from build123d import *

# Parameters (mm, degrees)
BOSS_EXTRUDE1_DEPTH   = 6
SKETCH3_W             = 7.6
SKETCH3_H             = 7.1
SKETCH3_H_2           = 14.9
CUT_EXTRUDE2_DEPTH    = 21.860671783
SKETCH4_W             = 7.6
SKETCH4_H             = 2.5
SKETCH4_W_2           = 5.5
SKETCH4_H_2           = 3.6
CUT_EXTRUDE3_DEPTH    = 21.860671783
FILLET2_R             = 3
F_2_56_TAPPED_HOLE1_D = 1.778
FILLET3_R             = 0.5
F_2_56_TAPPED_HOLE2_D = 1.778
SKETCH19_R            = 0.5
CUT_EXTRUDE6_DEPTH    = 21.860671783


with BuildPart() as part:
    # Sketch1 → Boss-Extrude1 (new body)
    with BuildSketch(Plane(origin=(7.5, 0, 0), x_dir=(0, 0, -1), z_dir=(1, 0, 0))):
        with BuildLine():
            Line((-10.5, 16.997577099), (-10.5, 5.397577099))
            Line((-10.5, 5.397577099), (-2, 5.397577099))
            Line((-2, 5.397577099), (-2, 15.497577099))
            ThreePointArc((-2, 15.497577099), (-1.5, 15.997577099), (-1, 15.497577099))
            Line((-1, 15.497577099), (-1, -2.902422901))
            Line((-1, -2.902422901), (7, -2.902422901))
            Line((7, -2.902422901), (7, 16.997577099))
            Line((7, 16.997577099), (-10.5, 16.997577099))
        make_face()
    extrude(amount=-BOSS_EXTRUDE1_DEPTH)

    # Sketch3 → Cut-Extrude2 (cut, through all)
    with BuildSketch(Plane.ZY.offset(-1.5)):
        with Locations((6.7, 13.947577099)):
            Rectangle(SKETCH3_W, SKETCH3_H)
        with Locations((-3.7, 10.047577099)):
            Rectangle(SKETCH3_W, SKETCH3_H_2)
    extrude(amount=-CUT_EXTRUDE2_DEPTH, mode=Mode.SUBTRACT)

    # Sketch4 → Cut-Extrude3 (cut, through all)
    with BuildSketch(Plane.ZY.offset(-1.5)):
        with Locations((6.7, 9.147577099)):
            Rectangle(SKETCH4_W, SKETCH4_H)
        with Locations((-4.736302331, 0.797577099)):
            Rectangle(SKETCH4_W_2, SKETCH4_H_2)
    extrude(amount=-CUT_EXTRUDE3_DEPTH, mode=Mode.SUBTRACT)

    # Fillet2
    fillet2_edges = [part.edges().sort_by_distance(p)[0] for p in [
        (1.5, 6.647577099, 10.5),
        (7.5, 6.647577099, 10.5),
        (7.5, -1.952422901, -7),
        (1.5, -1.952422901, -7),
    ]]
    fillet(fillet2_edges, radius=FILLET2_R - 0.0001)  # a hair under: the kernel refuses the full size

    # #2-56 Tapped Hole1 (through all)
    with Locations(Plane(origin=(0, 7.897577099, 0), x_dir=(1, 0, 0), z_dir=(0, 1, 0))):
        with Locations((4.5, -8)):
            Hole(F_2_56_TAPPED_HOLE1_D / 2)

    # Fillet3
    fillet3_edges = [part.edges().sort_by_distance(p)[0] for p in [
        (4.5, 2.597577099, 0.1),
        (4.5, 7.897577099, 2.9),
    ]]
    fillet(fillet3_edges, radius=FILLET3_R)

    # #2-56 Tapped Hole2 (through all)
    with Locations(Plane(origin=(0, -1.002422901, 0), x_dir=(1, 0, 0), z_dir=(0, 1, 0))):
        with Locations((4.5, 5)):
            Hole(F_2_56_TAPPED_HOLE2_D / 2)

    # Sketch19 → Cut-Extrude6 (cut, through all)
    with BuildSketch(Plane(origin=(7.5, 0, 0), x_dir=(0, 0, -1), z_dir=(1, 0, 0))):
        with Locations((2.269145043, -0.719580189)):
            Circle(SKETCH19_R)
    extrude(amount=-CUT_EXTRUDE6_DEPTH, mode=Mode.SUBTRACT)


solid = part.part
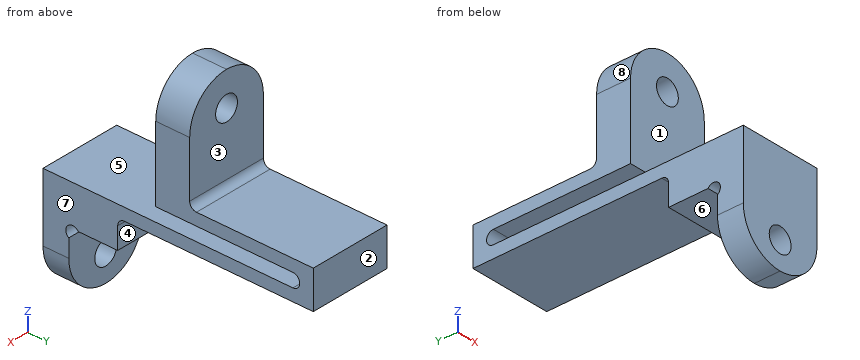
Build history of the part. All positions in model axes, mm. Face numbers are marked on the shaded views. A direction names the side the tool comes from. Round coordinates to 2 decimals unless told otherwise and drop trailing zeros. Write each loop counter-clockwise with the first axis right and the second up, starting at its lowest first coordinate (ties: lowest second). Pieces come first, ordered by that corner, then holes. Notation, with made-up numbers: (-16, 47) -> (-7, 47) arc R14 ccw to (-7, 70) -> close; hole circle Ø8 at (55, 65.25). An arc over 180 degrees is marked (long way). Use one line per item in the form item = value.
Q1. Drill centre lines: L1, parallel to Z at x = 4.5, y = 7.4; L2, parallel to Z at x = 5.5, y = 13; L3, parallel to Y at x = 1.85, z = 2.25. Where is each one in solid material? Low to high.
Conclusion:
L1 = 0.1 to 1, 2 to 7.11, 8.89 to 10.5
L2 = 0.1 to 1, 2 to 2.9
L3 = 5.4 to 17
Q2. Band-saw the part on A-A, the plane y = 7. State how many separate pieces and enclosed holes the cut face has, then the cut area to 3 significant figures.
Conclusion:
separate_pieces = 2
enclosed_holes = 1
area = 50.1 mm²
Q3. Band-saw the part on D-D, the plane y = 14. Write the cut outline in (x, z).
Conclusion:
outline = (1.5, 0.1) -> (7.5, 0.1) -> (7.5, 1) -> (1.5, 1) -> close; (1.5, 2) -> (7.5, 2) -> (7.5, 2.9) -> (1.5, 2.9) -> close
Q4. Tool access for the marked faces 1, 2, 3 and 4: list every direction of +Z, -Z, +X, -X, +Y, -Y with a clear straight run to the whole face (end or side of a thin tool).
Conclusion:
face_1 = +Z, +X, -X, -Y
face_2 = +Z, -Z, +X, -X, +Y
face_3 = +Z, +X, -X, +Y
face_4 = -Z, +X, -X, +Y
Q5. Band-saw the part on C-C, the plane x = 4. Write the cut outline in (y, z), then the cut area to 3 significant figures.
Conclusion:
outline = (-2.9, -6.96) -> (-1, -6.96) -> (-1, -5.74) -> (-2.9, -5.74) -> close; (-2.9, -4.26) -> (-1, -4.26) -> (-1, -2.68) arc R0.5 cw (long way) to (-0.31, -1.99) -> (2.6, -1.99) -> (2.6, -0.4) arc R0.5 cw to (3.1, 0.1) -> (17, 0.1) -> (17, 2.9) -> (8.4, 2.9) arc R0.5 cw to (7.9, 3.4) -> (7.9, 7.26) -> (5.4, 7.26) -> (5.4, 2) -> (15.5, 2) arc R0.5 cw to (15.5, 1) -> (-2.9, 1) -> close; (5.4, 8.74) -> (7.9, 8.74) -> (7.9, 10.46) -> (5.4, 10.46) -> close
area = 62.7 mm²
Q6. Drop flat-ended pins along their axis: P1, Ø3, axis at x = 4.5, y = 1.5, coming from the -Z side; P2, Ø1.4, axis at x = 4.5, z = 8, coming from the +Y side; P3, Ø1.8, axis at x = 4.5, y = 8.5, coming from the -Z side; P4, Ø1.8, axis at x = 3.5, y = 11.5, coming from the +Z side. Give the stop position or say it passes through.
Conclusion:
P1 = -1.99
P2 = through
P3 = 0.1
P4 = 2.9
Q7. Band-saw the part on B-B, the plane z = 8. Write the cut outline in (x, y).
Conclusion:
outline = (1.54, 5.4) -> (3.61, 5.4) -> (3.61, 7.9) -> (1.54, 7.9) -> close; (5.39, 5.4) -> (7.46, 5.4) -> (7.46, 7.9) -> (5.39, 7.9) -> close
Q8. Two-plate mould, pull along Z, no slides. Class the marked faces 5, 6, 7 and 8: released by +Z, released by -Z, zero draft, split by the parting line, or undercut.
Conclusion:
face_5 = undercut
face_6 = released by -Z
face_7 = zero draft
face_8 = released by +Z
